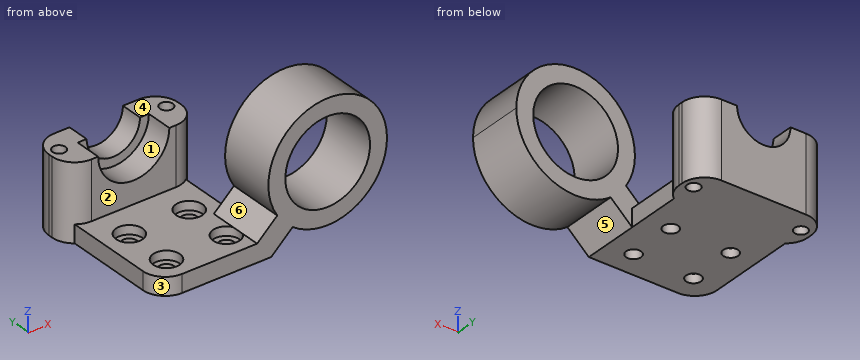
from build123d import *

# Parameters (mm, degrees)
F0_W      = 25
F0_H      = 35
F1_DEPTH  = 4
F2_R      = 1.675
F3_DEPTH  = 25
F4_W      = 25
F4_H      = 11
F5_DEPTH  = 13
F7_DEPTH  = 6
F8_R      = 8
F9_DEPTH  = 6
F2_R_2    = 3
F10_DEPTH = 2
F11_W     = 11
F11_H     = 17
F12_DEPTH = 2
F13_W     = 11
F13_H     = 17
F14_DEPTH = 2
F15_R     = 1.45
F16_DEPTH = 25
F17_R     = 5
F18_R     = 9.525
F19_DEPTH = 12.7
F20_R     = 5


with BuildPart() as f1:
    # F0 (on Top) → F1 (new body)
    with BuildSketch(Plane.XY):
        with Locations((12.5, 17.5)):
            Rectangle(F0_W, F0_H)
    extrude(amount=F1_DEPTH)

    # F2 (on face) → F3 (cut)
    with BuildSketch(Plane.XY.offset(4)):
        with BuildLine():
            ThreePointArc((4.094, 16.5088346784), (5.769, 14.8338346784), (7.444, 16.5088346784))
            ThreePointArc((7.444, 16.5088346784), (5.769, 18.1838346784), (4.094, 16.5088346784))
        make_face()
        with Locations((19.231, 16.5088346784)):
            Circle(F2_R)
        with Locations((19.231, 5.6122346784)):
            Circle(F2_R)
        with Locations((5.769, 5.6122346784)):
            Circle(F2_R)
    extrude(amount=-F3_DEPTH, mode=Mode.SUBTRACT)

    # F4 (on face) → F5 (join)
    with BuildSketch(Plane.XY.offset(4)):
        with Locations((12.5, 29.5)):
            Rectangle(F4_W, F4_H)
    extrude(amount=F5_DEPTH)

    # F6 (on face) → F7 (cut)
    with BuildSketch(Plane(origin=(0, 35, 0), x_dir=(-1, 0, 0), z_dir=(0, 1, 0))):
        with BuildLine():
            ThreePointArc((-18.5, 17), (-12.5, 11), (-6.5, 17))
            Line((-6.5, 17), (-18.5, 17))
        make_face()
    extrude(amount=-F7_DEPTH, mode=Mode.SUBTRACT)

    # F8 (on face) → F9 (cut)
    with BuildSketch(Plane.XZ.offset(-24)):
        with Locations((12.5, 17)):
            Circle(F8_R)
    extrude(amount=-F9_DEPTH, mode=Mode.SUBTRACT)

    # F2 (on face) → F10 (cut)
    with BuildSketch(Plane.XY.offset(4)):
        with BuildLine():
            ThreePointArc((8.769, 16.5088346784), (5.769, 19.5088346784), (2.769, 16.5088346784))
            ThreePointArc((2.769, 16.5088346784), (5.769, 13.5088346784), (8.769, 16.5088346784))
        make_face()
        with BuildLine():
            ThreePointArc((4.094, 16.5088346784), (5.769, 18.1838346784), (7.444, 16.5088346784))
            ThreePointArc((7.444, 16.5088346784), (5.769, 14.8338346784), (4.094, 16.5088346784))
        make_face(mode=Mode.SUBTRACT)
        with Locations((19.231, 16.5088346784)):
            Circle(F2_R_2)
        with Locations((19.231, 16.5088346784)):
            Circle(F2_R, mode=Mode.SUBTRACT)
        with Locations((19.231, 5.6122346784)):
            Circle(F2_R_2)
        with Locations((19.231, 5.6122346784)):
            Circle(F2_R, mode=Mode.SUBTRACT)
        with Locations((5.769, 5.6122346784)):
            Circle(F2_R_2)
        with Locations((5.769, 5.6122346784)):
            Circle(F2_R, mode=Mode.SUBTRACT)
    extrude(amount=-F10_DEPTH, mode=Mode.SUBTRACT)

    # F11 (on face) → F12 (join)
    with BuildSketch(Plane(origin=(0, 0, 0), x_dir=(0, -1, 0), z_dir=(-1, 0, 0))):
        with Locations((-29.5, 8.5)):
            Rectangle(F11_W, F11_H)
    extrude(amount=F12_DEPTH)

    # F13 (on face) → F14 (join)
    with BuildSketch(Plane.YZ.offset(25)):
        with Locations((29.5, 8.5)):
            Rectangle(F13_W, F13_H)
    extrude(amount=F14_DEPTH)

    # F15 (on face) → F16 (cut)
    with BuildSketch(Plane.XY.offset(17)):
        with Locations((0.4384, 30.174)):
            Circle(F15_R)
        with Locations((24.5616, 30.174)):
            Circle(F15_R)
    extrude(amount=-F16_DEPTH, mode=Mode.SUBTRACT)

    # F17
    f17_edges = [f1.edges().sort_by_distance(p)[0] for p in [
        (-2, 24, 8.5),
        (-2, 35, 8.5),
        (27, 35, 8.5),
        (27, 24, 8.5),
    ]]
    fillet(f17_edges, radius=F17_R)

    # F18 (on face) → F19 (join)
    with BuildSketch(Plane.XZ):
        with BuildLine():
            Line((26.3737617011, 8.2016371934), (29.8278119435, 4.4765953247))
            ThreePointArc((29.8278119435, 4.4765953247), (43.7351717982, 3.3488719473), (51.035, 15.24))
            ThreePointArc((51.035, 15.24), (34.0402980118, 28.0629796209), (26.3737617011, 8.2016371934))
        make_face()
        with Locations((37.7, 15.24)):
            Circle(F18_R, mode=Mode.SUBTRACT)
        with BuildLine():
            Line((25, 4), (25, 0))
            Line((25, 0), (29.8278119435, 4.4765953247))
            ThreePointArc((29.8278119435, 4.4765953247), (27.9217650948, 6.1731181138), (26.3737617011, 8.2016371934))
            Line((26.3737617011, 8.2016371934), (21.8424800567, 4))
            Line((21.8424800567, 4), (25, 4))
        make_face()
        with BuildLine():
            ThreePointArc((26.3737617011, 8.2016371934), (27.9217650948, 6.1731181138), (29.8278119435, 4.4765953247))
            Line((29.8278119435, 4.4765953247), (26.3737617011, 8.2016371934))
        make_face()
    extrude(amount=-F19_DEPTH)

    # F20
    f20_edges = [f1.edges().sort_by_distance(p)[0] for p in [
        (0, 0, 2),
    ]]
    fillet(f20_edges, radius=F20_R)


solid = f1.part
Build history of the part. All positions in model axes, mm. Face numbers are marked on the shaded views. A direction names the side the tool comes from. Round coordinates to 2 decimals unless told otherwise and drop trailing zeros. Loops run counter-clockwise (first coordinate to the right, second up) from the corner with the lowest first, then second, coordinate; pieces in that order, holes last. Notation, with made-up numbers: (0, 72) -> (5, 72) arc R19 ccw to (5, 103) -> close; hole circle Ø6 at (9, -30). An arc over 180 degrees is marked (long way). One line per item, written item: value. Start each with the question number.
Q1. Cut at A-A on x = 37.7. List the corners of the cut face in (y, z) (3 decimals).
Q2. Drop flat-ended pins along their axis: pin 1 Ø1.5 at (x, y) = (8, 27.5) entering from +Z; pin 2 Ø3 at (x, y) = (18.5, 5) entering from +Z; pin 3 Ø6 at (x, z) = (9, 17) entering from -Y. Give the stop position or say it passes through.
Q3. Probe line 1 along Y through (x, z) = (24, 4.75); line 2 along Y through (x, z) = (31.5, 27); line 3 along Z through (x, y) = (37.7, 4) (3 decimals). List the from-to ranges inside material, lowest first.
Q4. Cut at B-B on z = 16.25. List the corners of the cut face in (x, y), plus the area to 3 significant figures.
Q5. Cut at C-C on y = 15.5. List the corners of the cut face in (x, z).
Q6. Cut at D-D on x = 12.5. List the corners of the cut face in (y, z).
Q7. Two-plate mould, pull along X, no slides. Class the marked faces 1, 2 and 3: released by +X, released by -X, zero draft, split by the parting line, or undercut.
Q8. 3-axis set-ups, long thin cutter, end or side, ignore diameter. For the marked faces 4, 5 and 6: which of +Z, -Z, +X, -X, +Y, -Y reach the whole face in a straight line?
Computed:
1. outline: (0, 1.905) -> (12.7, 1.905) -> (12.7, 5.715) -> (0, 5.715) -> close; (0, 24.765) -> (12.7, 24.765) -> (12.7, 28.575) -> (0, 28.575) -> close
2. pin 1: z = 10.96
2. pin 2: z = 2
2. pin 3: y = 30
3. line 1: 0 to 12.7, 24.42 to 28.84, 31.51 to 34.58
3. line 2: 0 to 12.7
3. line 3: 1.905 to 5.715, 24.765 to 28.575
4. outline: (-2, 29) arc R5 ccw to (3, 24) -> (4.54, 24) -> (4.54, 30) -> (6.55, 30) -> (6.55, 35) -> (3, 35) arc R5 ccw to (-2, 30) -> close; (18.45, 30) -> (20.46, 30) -> (20.46, 24) -> (22, 24) arc R5 ccw to (27, 29) -> (27, 30) arc R5 ccw to (22, 35) -> (18.45, 35) -> close; (24.4, 0) -> (28.23, 0) -> (28.23, 12.7) -> (24.4, 12.7) -> close; (47.17, 0) -> (51, 0) -> (51, 12.7) -> (47.17, 12.7) -> close; hole circle Ø2.9 at (0.44, 30.17); hole circle Ø2.9 at (24.56, 30.17)
4. area: 226 mm²
5. outline: (0, 0) -> (4.43, 0) -> (4.43, 2) -> (2.94, 2) -> (2.94, 4) -> (0, 4) -> close; (7.11, 0) -> (17.89, 0) -> (17.89, 2) -> (16.41, 2) -> (16.41, 4) -> (8.59, 4) -> (8.59, 2) -> (7.11, 2) -> close; (20.57, 0) -> (25, 0) -> (25, 4) -> (22.06, 4) -> (22.06, 2) -> (20.57, 2) -> close
6. outline: (0, 0) -> (35, 0) -> (35, 11) -> (30, 11) -> (30, 9) -> (24, 9) -> (24, 4) -> (0, 4) -> close
7. face 1: undercut
7. face 2: zero draft
7. face 3: released by -X
8. face 4: +Z, +X, -X, +Y
8. face 5: -Z, -Y
8. face 6: -X, -Y
